Part model, mm, in its own coordinate system. A direction names the side the tool comes from. Give positions to 0.01 mm unless a question says otherwise; leave off trailing zeros. Loops run counter-clockwise (first coordinate to the right, second up) from the corner with the lowest first, then second, coordinate; pieces in that order, holes last. Notation, with made-up numbers: (31, 38.25) -> (42, 38.25) arc R21 ccw to (42, 54.25) -> close; hole circle Ø10 at (-13, -21.75). An arc over 180 degrees is marked (long way). Write item = value, one per line.
from build123d import *

# Parameters (mm, degrees)
EXTRUDE_1_DEPTH             = 80
EXTRUDE_2_DEPTH             = 4
EXTRUDE_START               = 4
EXTRUDE_3_DEPTH             = 4
CUT_EXTRUDE_1_DEPTH         = 4
CUT_EXTRUDE_2_REACH         = 176.531
SKETCH_5_R                  = 6.0000000000000036
CUT_EXTRUDE_START           = -4
CUT_EXTRUDE_3_DEPTH         = 4
SKETCH_7_R                  = 21
EXTRUDE_4_DEPTH             = 1
CUT_EXTRUDE_5_REACH         = 177.037
SKETCH_9_R                  = 4.599999999999999
SKETCH_9_R_2                = 1.3500000000000065
EXTRUDE_5_REACH             = 130.756
EXTRUDE_5_DIRECTION_2_REACH = 130.756
SKETCH_12_W                 = 138
SKETCH_12_H                 = 88
EXTRUDE_6_DEPTH             = 3
CHAMFER_1_SIZE              = 1
SKETCH_13_R                 = 2.5000000000000027
SKETCH_13_R_2               = 1.3999999999999955
SKETCH_13_R_3               = 2.5000000000000244
SKETCH_13_R_4               = 1.4000000000000308
EXTRUDE_7_DEPTH             = 45
FILLET_1_R                  = 4
FILLET_2_R                  = 4


with BuildPart() as part:
    # 草圖1 → 填料-伸長1 (new body)
    with BuildSketch(Plane.XY):
        with BuildLine():
            Line((-4, -1.6620202496294076), (-4, 54.00000000000001))
            Line((-4, 54.00000000000001), (134, 54.00000000000001))
            Line((134, 54.00000000000001), (134, -1.662020249629414))
            Line((134, -1.662020249629414), (98.96497064934022, -36.54297400803102))
            ThreePointArc((98.96497064934022, -36.54297400803102), (65.00000000000001, -69), (31.035029350659826, -36.54297400803101))
            Line((31.035029350659826, -36.54297400803101), (-4, -1.6620202496294076))
        make_face()
        with BuildLine():
            Line((0, 0), (0, 50))
            Line((0, 50), (130, 50))
            Line((130, 50), (130, 0))
            Line((130, 0), (94.99960713766303, -34.8464695929839))
            ThreePointArc((94.99960713766303, -34.8464695929839), (65.00000000000001, -65), (35.000392862337, -34.84646959298392))
            Line((35.000392862337, -34.84646959298392), (0, 0))
        make_face(mode=Mode.SUBTRACT)
    extrude(amount=EXTRUDE_1_DEPTH)

    # 草圖2 → 填料-伸長2 (add)
    # profile 1 of 2: a face of its own
    with BuildSketch(Plane.XY.offset(80)):
        with BuildLine():
            Line((-4, 54.00000000000001), (-4, -1.6620202496294076))
            Line((-4, -1.6620202496294076), (31.03502935065982, -36.54297400803101))
            ThreePointArc((31.03502935065982, -36.54297400803101), (65.00000000000001, -69), (98.96497064934022, -36.54297400803102))
            Line((98.96497064934022, -36.54297400803102), (134, -1.662020249629414))
            Line((134, -1.662020249629414), (134, 54.00000000000001))
            Line((134, 54.00000000000001), (-4, 54.00000000000001))
        make_face()
        with BuildLine():
            Line((130, 0), (94.99960713766303, -34.8464695929839))
            ThreePointArc((94.99960713766303, -34.8464695929839), (65.00000000000003, -65), (35.000392862337, -34.84646959298392))
            Line((35.000392862337, -34.84646959298392), (0, 0))
            Line((0, 0), (0, 50))
            Line((0, 50), (130, 50))
            Line((130, 50), (130, 0))
        make_face(mode=Mode.SUBTRACT)
    # profile 2 of 2: a face of its own
    with BuildSketch(Plane.XY.offset(80)):
        with BuildLine():
            ThreePointArc((94.99960713766303, -34.8464695929839), (65.00000000000003, -65), (35.000392862337, -34.84646959298392))
            Line((35.000392862337, -34.84646959298392), (0, 0))
            Line((0, 0), (0, 50))
            Line((0, 50), (130, 50))
            Line((130, 50), (130, 0))
            Line((130, 0), (94.99960713766303, -34.8464695929839))
        make_face()
    extrude(amount=EXTRUDE_2_DEPTH)

    # 草圖3 → 填料-伸長3 (add)
    with BuildSketch(Plane(origin=(0, 0, 0), x_dir=(-1, 0, 0), z_dir=(0, 0, -1)).offset(EXTRUDE_START)):
        with BuildLine():
            Line((-134, 54.00000000000001), (-134, -1.662020249629414))
            Line((-134, -1.662020249629414), (-98.9649706493402, -36.54297400803101))
            ThreePointArc((-98.9649706493402, -36.54297400803101), (-65.00000000000001, -69), (-31.03502935065982, -36.54297400803101))
            Line((-31.03502935065982, -36.54297400803101), (4, -1.6620202496294076))
            Line((4, -1.6620202496294076), (4, 54.00000000000001))
            Line((4, 54.00000000000001), (-134, 54.00000000000001))
        make_face()
    extrude(amount=-EXTRUDE_3_DEPTH)

    # 草圖4 → 除料-伸長1 (cut)
    with BuildSketch(Plane(origin=(0, 54.00000000000001, 0), x_dir=(1, 0, 0), z_dir=(0, 1, 0))):
        Polygon((0, 1.73e-15), (130, 0), (130, -80), (1.029e-14, -80), align=None)
    extrude(amount=-CUT_EXTRUDE_1_DEPTH, mode=Mode.SUBTRACT)

    # 除料-伸長2: up to this face of the body (flat: up to its plane)
    cut_extrude_2_end = Plane(part.part.faces().sort_by_distance((65, 4.120950098, -4))[0])
    # 草圖5 → 除料-伸長2 (cut, up to the picked face)
    with BuildSketch(Plane.XY.offset(84), mode=Mode.PRIVATE) as cut_extrude_2_sk1:
        with Locations((65.00000000000001, -35)):
            Circle(SKETCH_5_R)
    cut_extrude_2_tool1 = split(extrude(cut_extrude_2_sk1.sketch, amount=-CUT_EXTRUDE_2_REACH, mode=Mode.PRIVATE), bisect_by=cut_extrude_2_end, keep=Keep.BOTH, mode=Mode.PRIVATE)
    add(cut_extrude_2_tool1.solids().sort_by(Axis((65, -35, 84), (0, 0, -1)))[0], mode=Mode.SUBTRACT)

    # 草圖6 → 除料-伸長3 (cut)
    with BuildSketch(Plane.XY.offset(84).offset(CUT_EXTRUDE_START)):
        with BuildLine():
            ThreePointArc((64.99999999999967, -45), (60.77381738259285, -44.06307787036642), (57.33955556881022, -41.427876096865376))
            Line((57.339555568810226, -41.42787609686538), (42.01866670643064, -54.28362829059615))
            ThreePointArc((42.01866670643065, -54.28362829059614), (52.32145214777887, -62.18923361109942), (64.99999999999969, -65))
            Line((65.00000000000004, -65), (65.00000000000003, -45.00000000000001))
        make_face()
        with BuildLine():
            Line((87.9813332935694, -54.28362829059614), (72.66044443118982, -41.427876096865376))
            ThreePointArc((72.66044443118982, -41.427876096865376), (69.22618261740686, -44.06307787036657), (64.99999999999967, -45))
            Line((65.00000000000003, -45.00000000000001), (65.00000000000004, -65))
            ThreePointArc((64.99999999999969, -65), (77.67854785222087, -62.18923361109955), (87.9813332935694, -54.28362829059614))
        make_face()
    extrude(amount=CUT_EXTRUDE_3_DEPTH, mode=Mode.SUBTRACT)

    # 草圖7 → 填料-伸長4 (add)
    with BuildSketch(Plane(origin=(0, 0, -4), x_dir=(-1, 0, 0), z_dir=(0, 0, -1))):
        with Locations((-65.00000000000001, -43)):
            Circle(SKETCH_7_R)
    extrude(amount=EXTRUDE_4_DEPTH)

    # 草圖9 → 除料-伸長5 (cut, up to next)
    with BuildSketch(Plane(origin=(0, 0, -5), x_dir=(-1, 0, 0), z_dir=(0, 0, -1)), mode=Mode.PRIVATE) as cut_extrude_5_sk1:
        with Locations((-65.00000000000001, -35)):
            Circle(SKETCH_9_R)
    cut_extrude_5_tool1 = extrude(cut_extrude_5_sk1.sketch, amount=-CUT_EXTRUDE_5_REACH, mode=Mode.PRIVATE) & part.part
    # 草圖9 → 除料-伸長5 (cut, up to next)
    with BuildSketch(Plane(origin=(0, 0, -5), x_dir=(-1, 0, 0), z_dir=(0, 0, -1)), mode=Mode.PRIVATE) as cut_extrude_5_sk2:
        with Locations((-82.50000000000001, -43)):
            Circle(SKETCH_9_R_2)
    cut_extrude_5_tool2 = extrude(cut_extrude_5_sk2.sketch, amount=-CUT_EXTRUDE_5_REACH, mode=Mode.PRIVATE) & part.part
    # 草圖9 → 除料-伸長5 (cut, up to next)
    with BuildSketch(Plane(origin=(0, 0, -5), x_dir=(-1, 0, 0), z_dir=(0, 0, -1)), mode=Mode.PRIVATE) as cut_extrude_5_sk3:
        with Locations((-47.50000000000001, -43)):
            Circle(SKETCH_9_R_2)
    cut_extrude_5_tool3 = extrude(cut_extrude_5_sk3.sketch, amount=-CUT_EXTRUDE_5_REACH, mode=Mode.PRIVATE) & part.part
    add(cut_extrude_5_tool1.solids().sort_by_distance((65, -35, -5))[0], mode=Mode.SUBTRACT)
    add(cut_extrude_5_tool2.solids().sort_by_distance((82.5, -43, -5))[0], mode=Mode.SUBTRACT)
    add(cut_extrude_5_tool3.solids().sort_by_distance((47.5, -43, -5))[0], mode=Mode.SUBTRACT)

    # 填料-伸長5: up to this face of the body (flat: up to its plane)
    extrude_5_end = Plane(part.part.faces().sort_by_distance((130, 27, 40))[0])
    # 草圖10 → 填料-伸長5 (add, up to the picked face)
    with BuildSketch(Plane(origin=(65, 0, 0), x_dir=(0, 0, -1), z_dir=(1, 0, 0)), mode=Mode.PRIVATE) as extrude_5_sk1:
        Polygon((-83, 26.160223806036317), (-60.34563272960637, 1.0000000000000073), (-59.00000000000001, 1.0000000000000078), (-84, 28.765312870730142), (-84, 1.0000000000000044), (-83, 1.0000000000000044), align=None)
    extrude_5_tool1 = split(extrude(extrude_5_sk1.sketch, amount=EXTRUDE_5_REACH, mode=Mode.PRIVATE), bisect_by=extrude_5_end, keep=Keep.BOTH, mode=Mode.PRIVATE)
    add(extrude_5_tool1.solids().sort_by(Axis((65, 13.830112, 71.395163), (1, 0, 0)))[0])

    # 填料-伸長5 direction 2: up to this face of the body (flat: up to its plane)
    extrude_5_direction_2_end = Plane(part.part.faces().sort_by_distance((0, 27, 40))[0])
    # 草圖10 → 填料-伸長5 direction 2 (add, up to the picked face)
    with BuildSketch(Plane(origin=(65, 0, 0), x_dir=(0, 0, -1), z_dir=(1, 0, 0)), mode=Mode.PRIVATE) as extrude_5_direction_2_sk1:
        Polygon((-83, 26.160223806036317), (-60.34563272960637, 1.0000000000000073), (-59.00000000000001, 1.0000000000000078), (-84, 28.765312870730142), (-84, 1.0000000000000044), (-83, 1.0000000000000044), align=None)
    extrude_5_direction_2_tool1 = split(extrude(extrude_5_direction_2_sk1.sketch, amount=-EXTRUDE_5_DIRECTION_2_REACH, mode=Mode.PRIVATE), bisect_by=extrude_5_direction_2_end, keep=Keep.BOTH, mode=Mode.PRIVATE)
    add(extrude_5_direction_2_tool1.solids().sort_by(Axis((65, 13.830112, 71.395163), (-1, 0, 0)))[0])

    # 草圖12 → 填料-伸長6 (add)
    with BuildSketch(Plane(origin=(0, 54.00000000000001, 0), x_dir=(1, 0, 0), z_dir=(0, 1, 0))):
        Polygon((-6, 6), (136, 6), (136, -86), (-5.9999999999999885, -86), align=None)
        with Locations((65, -40)):
            Rectangle(SKETCH_12_W, SKETCH_12_H, mode=Mode.SUBTRACT)
    extrude(amount=-EXTRUDE_6_DEPTH)

    # 導角1
    chamfer_1_edges = [part.edges().sort_by_distance(p)[0] for p in [
        (86.00000000000001, -43, -4),
    ]]
    chamfer(chamfer_1_edges, length=CHAMFER_1_SIZE - 0.0001)  # a hair under: the kernel refuses the full size

    # 草圖13 → 填料-伸長7 (add)
    # profile 1 of 2: a face of its own
    with BuildSketch(Plane.XY.offset(84)):
        with Locations((29.000000000000018, -36.54297400803102)):
            Circle(SKETCH_13_R)
        with Locations((29.000000000000018, -36.54297400803102)):
            Circle(SKETCH_13_R_2, mode=Mode.SUBTRACT)
    # profile 2 of 2: a face of its own
    with BuildSketch(Plane.XY.offset(84)):
        with Locations((101, -36.54297400803102)):
            Circle(SKETCH_13_R_3)
        with Locations((101, -36.54297400803102)):
            Circle(SKETCH_13_R_4, mode=Mode.SUBTRACT)
    extrude(amount=-EXTRUDE_7_DEPTH)

    # 圓角1
    fillet_1_edges = [part.edges().sort_by_distance(p)[0] for p in [
        (42.01866670643065, -54.28362829059614, 82),
        (87.9813332935694, -54.28362829059614, 82),
    ]]
    fillet(fillet_1_edges, radius=FILLET_1_R)

    # 圓角2
    fillet_2_edges = [part.edges().sort_by_distance(p)[0] for p in [
        (31.121034817860412, -37.86630741327102, 61.5),
        (98.87896518213962, -37.86630741327102, 61.5),
    ]]
    fillet(fillet_2_edges, radius=FILLET_2_R)


solid = part.part
1) Drill centre lines: line 1 along X through (y, z) = (19.5, 67.5); line 2 along Z through (x, y) = (50, 0); line 3 along Y through (x, z) = (65, -0.85). Where is each one in solid material? Low to high. Write a range as [from, to].
Resolved:
line_1 = [-4, 0], [130, 134]
line_2 = [-4, 0], [80, 84]
line_3 = [-69, -41], [-29, 54]
2) Slice it at C-C, the plane x = 89.5. List the corners of the cut face in (y, z).
Resolved:
outline = (-58.57, -4) -> (51, -4) -> (51, -6) -> (54, -6) -> (54, 0) -> (-52.31, 0) -> (-52.31, 80) -> (22.83, 80) -> (1, 60.35) -> (1, 59) -> (24.32, 80) -> (54, 80) -> (54, 86) -> (51, 86) -> (51, 84) -> (-58.57, 84) -> close
3) Slice it at B-B, the plane z = 26. List the corners of the cut face in (x, y).
Resolved:
outline = (-6, 51) -> (-4, 51) -> (-4, -1.66) -> (31.04, -36.54) arc R34 ccw to (98.96, -36.54) -> (134, -1.66) -> (134, 51) -> (136, 51) -> (136, 54) -> (130, 54) -> (130, 0) -> (95, -34.85) arc R30 cw (long way) to (35, -34.85) -> (0, 0) -> (0, 54) -> (-6, 54) -> close
4) Which spindle directions (+Z, -Z, +X, -X, +Y, -Y) get a long thin tool onto all of the face, cutting with end or side? Do faces 4 (the face through (17.75, -17.67, 39.44)), 5 (the face through (64, 9, 0)), 6 (the face through (68.65, -37.8, -4.51)), 7 (the face through (86.108, -54.489, 82.028)). Say none if no direction does.
Resolved:
face_4 = none
face_5 = +Y
face_6 = +Z, -Z
face_7 = +Z
5) Drop flat-ended pins along their axis: P1, Ø2, axis at x = 29, y = -36.54, coming from the +Z side; P2, Ø12.5, axis at x = 60.5, y = -38, coming from the -Z side; P3, Ø15, axis at x = 77.5, y = 43, coming from the -Z side; P4, Ø15.5, axis at x = 65, y = -35, coming from the +Z side. Give the stop position or say it passes through.
Resolved:
P1 = through
P2 = -5
P3 = -4
P4 = 84
6) Pull direction Z, two halves, no side cores. Call faces 1 (the face through (66, -8, 80)), 2 (the face through (28.9, -38.1, 39)), 3 (the face through (65, 51, -5)): pulls with the +Z half, pulls with the -Z half, needs draft (parallel to the pull), parting line crosses it, or undercut.
Resolved:
face_1 = undercut
face_2 = pulls with the -Z half
face_3 = needs draft
7) Slice it at A-A, the plane y = 13.5. List the corners of the cut face in (x, z).
Resolved:
outline = (-4, -4) -> (134, -4) -> (134, 84) -> (-4, 84) -> close; hole (0, 0) -> (130, 0) -> (130, 70.26) -> (0, 70.26) -> close; hole (0, 71.6) -> (130, 71.6) -> (130, 80) -> (0, 80) -> close
8) Slice it at D-D, the plane x = 65. Count the separate pieces of the cut face and the enclosed holes in it, and give its area (3 significant figures).
Resolved:
separate_pieces = 4
enclosed_holes = 0
area = 1,200 mm²
